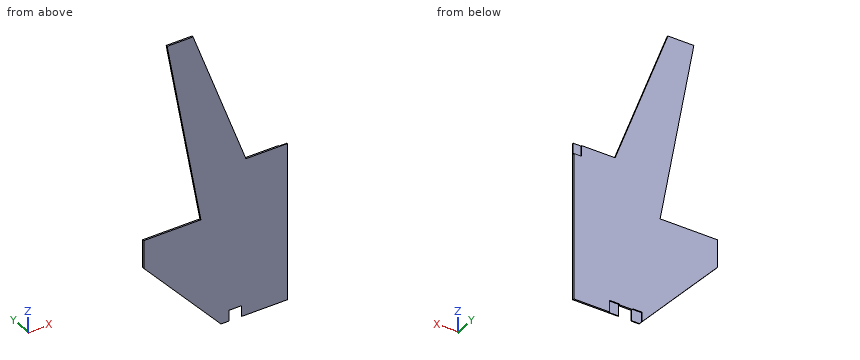
```python
from build123d import *

# Parameters (mm, degrees)
F0_W     = 45
F0_H     = 62
F1_DEPTH = 9
F2_DEPTH = 5


with BuildPart() as f1:
    # F0 (on Front) → F1 (new body)
    with BuildSketch(Plane.XZ):
        Polygon((-435.104496, 482.891372), (-11, 12.208114), (-11, 67), (44, 67), (44, 62), (117, 62), (117, 67), (172, 67), (172, 0), (373.629411, 0), (373.629411, 838), (328.629411, 838), (328.629411, 900), (140.629411, 900), (-157.3519, 1713.119388), (-303.3519, 1713.119388), (-113.104496, 642.891372), (-435.104496, 642.891372), align=None)
        Polygon((-11, 12.208114), (0, 0), (44, 0), (44, 62), (44, 67), (-11, 67), align=None)
        Polygon((117, 67), (117, 62), (117, 0), (172, 0), (172, 67), align=None)
        with Locations((351.129411, 869)):
            Rectangle(F0_W, F0_H)
    extrude(amount=F1_DEPTH)

    # F0 (on Front) → F2 (cut)
    with BuildSketch(Plane.XZ):
        with Locations((351.129411, 869)):
            Rectangle(F0_W, F0_H)
        Polygon((-11, 12.208114), (0, 0), (44, 0), (44, 62), (44, 67), (-11, 67), align=None)
        Polygon((117, 67), (117, 62), (117, 0), (172, 0), (172, 67), align=None)
    extrude(amount=F2_DEPTH, mode=Mode.SUBTRACT)


solid = f1.part
```
Geometry: final body of the model. Coordinates: model frame, mm. Coordinates: 2 decimals unless noted, no trailing zeros. Order: outer loops, then holes, each group sorted by start corner. A loop starts at its lowest first (then second) coordinate and runs counter-clockwise, first axis right, second up. Notation, with made-up numbers: (-38.75, 88) - (6.25, 88) arc R7 ccw to (6.25, 99) - close; hole circle Ø9 at (29.5, 29). An arc over 180 degrees is marked (long way). Write each question's results on one line, items separated by ' | '.
1) Pin query (flat end, axial travel): pin 1 (4 mm diameter, centred on x = -44.5, y = -5.5, fed in from -Z); pin 2 (1.5 mm diameter, centred on y = -3, z = 884, fed in from +X); pin 3 (4 mm diameter, centred on y = -3.5, z = 27.5, fed in from -X). Return the tip coordinate at first contact, or that it passes through.
Results list:
pin 1: z = 47.17 | pin 2: x = 328.63 | pin 3: x = -26.58
2) Section C-C, the plane x = 199. Return loops of the section in (y, z).
Results list:
outline: (-9, 0) - (0, 0) - (0, 900) - (-9, 900) - close
3) Line query: line 1 (Z direction, x = 184, y = -4); line 2 (X direction, y = -0.75, z = 1429.5); line 3 (X direction, y = -7, z = 699.5). Output: solid intervals per line, ascending. Write a range as from..to.
Results list:
line 1: 0..900 | line 2: -252.93..-53.41 | line 3: -123.17..373.63
4) Section B-B, the plane x = -238. Return loops of the section in (y, z), plus the area to 3 significant figures.
Results list:
outline: (-9, 264.14) - (0, 264.14) - (0, 642.89) - (-9, 642.89) - close; (-9, 1345.49) - (0, 1345.49) - (0, 1713.12) - (-9, 1713.12) - close | area: 6,720 mm^2
5) Section D-D, the plane z = 1156. Return loops of the section in (x, y), plus the area to 3 significant figures.
Results list:
outline: (-204.32, -9) - (46.81, -9) - (46.81, 0) - (-204.32, 0) - close | area: 2,260 mm^2
6) Section A-A, the plane y = -2.5. Return loops of the section in (x, z), plus the area to 3 significant figures.
Results list:
outline: (-435.1, 482.89) - (-11, 12.21) - (-11, 67) - (44, 67) - (44, 62) - (117, 62) - (117, 67) - (172, 67) - (172, 0) - (373.63, 0) - (373.63, 838) - (328.63, 838) - (328.63, 900) - (140.63, 900) - (-157.35, 1713.12) - (-303.35, 1713.12) - (-113.1, 642.89) - (-435.1, 642.89) - close | area: 712,000 mm^2
